Design review of the part built by this model. Coordinates are the model's own, in mm. Face numbers are marked on the shaded views. A direction names the side the tool comes from. Coordinates: 2 decimals unless noted, no trailing zeros. Order: outer loops, then holes, each group sorted by start corner. A loop starts at its lowest first (then second) coordinate and runs counter-clockwise, first axis right, second up.
from build123d import *

# Parameters (mm, degrees)
F0_W      = 9
F0_H      = 9
F1_DEPTH  = 4
F7_DEPTH  = 3.375
F8_DEPTH  = 3.375
F9_DEPTH  = 3.375
F10_DEPTH = 3.375
F11_D     = 13.25


with BuildPart() as f1:
    # F0 (on Top) → F1 (new body)
    with BuildSketch(Plane.XY):
        with BuildLine():
            ThreePointArc((4.5, -14.8323969742), (0, -15.5), (-4.5, -14.8323969742))
            Line((-4.5, -14.8323969742), (-4.5, -44.4))
            Line((-4.5, -44.4), (4.5, -44.4))
            Line((4.5, -44.4), (4.5, -14.8323969742))
        make_face()
        with BuildLine():
            Line((4.5, -4.5), (-4.5, -4.5))
            Line((-4.5, -4.5), (-4.5, -14.8323969742))
            ThreePointArc((-4.5, -14.8323969742), (0, -15.5), (4.5, -14.8323969742))
            Line((4.5, -14.8323969742), (4.5, -4.5))
        make_face()
        with BuildLine():
            Line((-4.5, -4.5), (-14.8323969742, -4.5))
            ThreePointArc((-14.8323969742, -4.5), (-10.9601551084, -10.9601551084), (-4.5, -14.8323969742))
            Line((-4.5, -14.8323969742), (-4.5, -4.5))
        make_face()
        with BuildLine():
            Line((-4.5, 4.5), (-14.8323969742, 4.5))
            ThreePointArc((-14.8323969742, 4.5), (-15.5, 0), (-14.8323969742, -4.5))
            Line((-14.8323969742, -4.5), (-4.5, -4.5))
            Line((-4.5, -4.5), (-4.5, 4.5))
        make_face()
        with BuildLine():
            Line((14.8323969742, -4.5), (4.5, -4.5))
            Line((4.5, -4.5), (4.5, -14.8323969742))
            ThreePointArc((4.5, -14.8323969742), (10.9601551084, -10.9601551084), (14.8323969742, -4.5))
        make_face()
        with BuildLine():
            Line((14.8323969742, 4.5), (4.5, 4.5))
            Line((4.5, 4.5), (4.5, -4.5))
            Line((4.5, -4.5), (14.8323969742, -4.5))
            ThreePointArc((14.8323969742, -4.5), (15.3321908594, -2.2746260022), (15.5, 0))
            ThreePointArc((15.5, 0), (15.3321908594, 2.2746260022), (14.8323969742, 4.5))
        make_face()
        with BuildLine():
            Line((44.4, 4.5), (14.8323969742, 4.5))
            ThreePointArc((14.8323969742, 4.5), (15.3321908594, 2.2746260022), (15.5, 0))
            ThreePointArc((15.5, 0), (15.3321908594, -2.2746260022), (14.8323969742, -4.5))
            Line((14.8323969742, -4.5), (44.4, -4.5))
            Line((44.4, -4.5), (44.4, 4.5))
        make_face()
        with BuildLine():
            Line((-14.8323969742, 4.5), (-44.4, 4.5))
            Line((-44.4, 4.5), (-44.4, -4.5))
            Line((-44.4, -4.5), (-14.8323969742, -4.5))
            ThreePointArc((-14.8323969742, -4.5), (-15.5, 0), (-14.8323969742, 4.5))
        make_face()
        Rectangle(F0_W, F0_H)
        with BuildLine():
            Line((-4.5, 14.8323969742), (-4.5, 4.5))
            Line((-4.5, 4.5), (4.5, 4.5))
            Line((4.5, 4.5), (4.5, 14.8323969742))
            ThreePointArc((4.5, 14.8323969742), (0, 15.5), (-4.5, 14.8323969742))
        make_face()
        with BuildLine():
            Line((4.5, 14.8323969742), (4.5, 4.5))
            Line((4.5, 4.5), (14.8323969742, 4.5))
            ThreePointArc((14.8323969742, 4.5), (10.9601551084, 10.9601551084), (4.5, 14.8323969742))
        make_face()
        with BuildLine():
            Line((-4.5, 44.4), (-4.5, 14.8323969742))
            ThreePointArc((-4.5, 14.8323969742), (0, 15.5), (4.5, 14.8323969742))
            Line((4.5, 14.8323969742), (4.5, 44.4))
            Line((4.5, 44.4), (-4.5, 44.4))
        make_face()
        with BuildLine():
            ThreePointArc((-4.5, 14.8323969742), (-10.9601551084, 10.9601551084), (-14.8323969742, 4.5))
            Line((-14.8323969742, 4.5), (-4.5, 4.5))
            Line((-4.5, 4.5), (-4.5, 14.8323969742))
        make_face()
    extrude(amount=F1_DEPTH)

    # F3 (on face) → F7 (join)
    with BuildSketch(Plane.XZ.offset(44.4)):
        with BuildLine():
            Line((4.5, 0), (-4.5, 0))
            Line((-4.5, 0), (-4.5, -3))
            ThreePointArc((-4.5, -3), (0, -1.5), (4.5, -3))
            Line((4.5, -3), (4.5, 0))
        make_face()
        with BuildLine():
            Line((4.5, -3), (-4.5, -3))
            ThreePointArc((-4.5, -3), (-7.4938552368, -9.3035353181), (-4, -15.3442887702))
            Line((-4, -15.3442887702), (-2.5, -10.4197270865))
            ThreePointArc((-2.5, -10.4197270865), (-0.7342087578, -6.2203305053), (2.875, -9))
            ThreePointArc((2.875, -9), (2.7796694947, -9.7342087578), (2.5, -10.4197270865))
            Line((2.5, -10.4197270865), (4, -15.3442887702))
            ThreePointArc((4, -15.3442887702), (6.5669627683, -12.6228441865), (7.5, -9))
            ThreePointArc((7.5, -9), (6.7082039325, -5.6458980338), (4.5, -3))
        make_face()
        with BuildLine():
            ThreePointArc((4.5, -3), (0, -1.5), (-4.5, -3))
            Line((-4.5, -3), (4.5, -3))
        make_face()
    extrude(amount=-F7_DEPTH)

    # F6 (on face) → F8 (join)
    with BuildSketch(Plane.YZ.offset(44.4)):
        with BuildLine():
            Line((4.5, 0), (-4.5, 0))
            Line((-4.5, 0), (-4.5, -3))
            ThreePointArc((-4.5, -3), (0, -1.5), (4.5, -3))
            Line((4.5, -3), (4.5, 0))
        make_face()
        with BuildLine():
            ThreePointArc((4.5, -3), (0, -1.5), (-4.5, -3))
            Line((-4.5, -3), (4.5, -3))
        make_face()
        with BuildLine():
            Line((4.5, -3), (-4.5, -3))
            ThreePointArc((-4.5, -3), (-7.4938552368, -9.3035353181), (-4, -15.3442887702))
            Line((-4, -15.3442887702), (-2.5, -10.4197270865))
            ThreePointArc((-2.5, -10.4197270865), (-0.7342087578, -6.2203305053), (2.875, -9))
            ThreePointArc((2.875, -9), (2.7796694947, -9.7342087578), (2.5, -10.4197270865))
            Line((2.5, -10.4197270865), (4, -15.3442887702))
            ThreePointArc((4, -15.3442887702), (6.5669627683, -12.6228441865), (7.5, -9))
            ThreePointArc((7.5, -9), (6.7082039325, -5.6458980338), (4.5, -3))
        make_face()
    extrude(amount=-F8_DEPTH)

    # F5 (on face) → F9 (join)
    with BuildSketch(Plane(origin=(0, 44.4, 0), x_dir=(-1, 0, 0), z_dir=(0, 1, 0))):
        with BuildLine():
            Line((4.5, 0), (-4.5, 0))
            Line((-4.5, 0), (-4.5, -3))
            ThreePointArc((-4.5, -3), (0, -1.5), (4.5, -3))
            Line((4.5, -3), (4.5, 0))
        make_face()
        with BuildLine():
            ThreePointArc((4.5, -3), (0, -1.5), (-4.5, -3))
            Line((-4.5, -3), (4.5, -3))
        make_face()
        with BuildLine():
            Line((4.5, -3), (-4.5, -3))
            ThreePointArc((-4.5, -3), (-7.4938552368, -9.3035353181), (-4, -15.3442887702))
            Line((-4, -15.3442887702), (-2.5, -10.4197270865))
            ThreePointArc((-2.5, -10.4197270865), (-0.7342087578, -6.2203305053), (2.875, -9))
            ThreePointArc((2.875, -9), (2.7796694947, -9.7342087578), (2.5, -10.4197270865))
            Line((2.5, -10.4197270865), (4, -15.3442887702))
            ThreePointArc((4, -15.3442887702), (6.5669627683, -12.6228441865), (7.5, -9))
            ThreePointArc((7.5, -9), (6.7082039325, -5.6458980338), (4.5, -3))
        make_face()
    extrude(amount=-F9_DEPTH)

    # F4 (on face) → F10 (join)
    with BuildSketch(Plane(origin=(-44.4, 0, 0), x_dir=(0, -1, 0), z_dir=(-1, 0, 0))):
        with BuildLine():
            Line((4.5, 0), (-4.5, 0))
            Line((-4.5, 0), (-4.5, -3))
            ThreePointArc((-4.5, -3), (0, -1.5), (4.5, -3))
            Line((4.5, -3), (4.5, 0))
        make_face()
        with BuildLine():
            Line((4.5, -3), (-4.5, -3))
            ThreePointArc((-4.5, -3), (-7.4938552368, -9.3035353181), (-4, -15.3442887702))
            Line((-4, -15.3442887702), (-2.5, -10.4197270865))
            ThreePointArc((-2.5, -10.4197270865), (-0.7342087578, -6.2203305053), (2.875, -9))
            ThreePointArc((2.875, -9), (2.7796694947, -9.7342087578), (2.5, -10.4197270865))
            Line((2.5, -10.4197270865), (4, -15.3442887702))
            ThreePointArc((4, -15.3442887702), (6.5669627683, -12.6228441865), (7.5, -9))
            ThreePointArc((7.5, -9), (6.7082039325, -5.6458980338), (4.5, -3))
        make_face()
        with BuildLine():
            ThreePointArc((4.5, -3), (0, -1.5), (-4.5, -3))
            Line((-4.5, -3), (4.5, -3))
        make_face()
    extrude(amount=-F10_DEPTH)

    # F11 (through all)
    with Locations(Plane(origin=(0, 0, 0), x_dir=(1, 0, 0), z_dir=(0, 0, -1))):
        with Locations((0, 0)):
            Hole(F11_D / 2)


solid = f1.part
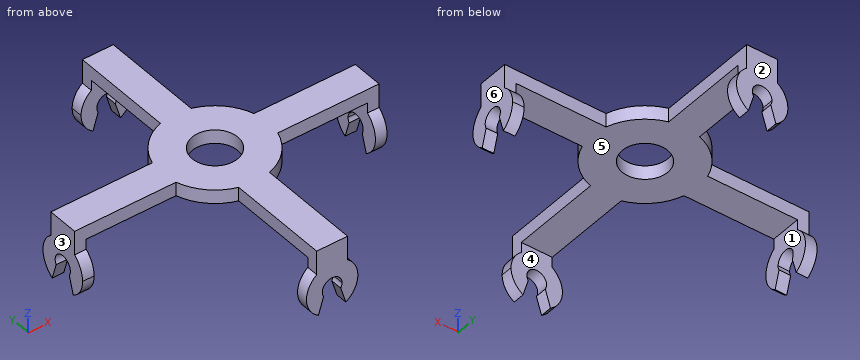
1. Mouldability with a two-part tool opening along X and no side actions: class the marked faces 1, 2 and 3 as pulls with the +X half, pulls with the -X half, needs draft (parallel to the pull), parting line crosses it, or undercut.
2. Add section A-A (y = 0). Give the boundary of the cut face in (x, z) (3 decimals), and give its area (3 significant figures).
3. For the marked faces 4, 5 and 6, list the 3-axis set-ups (+Z, -Z, +X, -X, +Y, -Y) from which the entire face can be reached by the end or side of a thin tool; tool diameter is ignored.
4. Add section D-D (x = 24.5). Give the boundary of the cut face in (y, z).
5. To check wall thickness, follow line 1 (Y direction, x = 7, z = -10.5) (3 decimals); line 2 (Y direction, x = -42.8, z = -9) (3 decimals). State the ranges of each line that lie inside material, in increasing order.
6. Insertion check: pin 1 (5.5 mm diameter, centred on y = -34.5, z = -0.5, fed in from -X); pin 2 (7.5 mm diameter, centred on y = 30, z = 2, fed in from +X); pin 3 (2 mm diameter, centred on y = -12.5, z = -2.5, fed in from +X); pin 4 (3.5 mm diameter, centred on x = 33, z = 1.5, fed in from -Y). Each pin has a flat end and moves straight along its axis. Give the tip position at first contact, or say it passes through.
7. Add section C-C (z = -12). State how many separate pieces and enclosed holes the cut face has, and give its area (3 significant figures).
Solution:
1. face 1: undercut
1. face 2: needs draft
1. face 3: pulls with the -X half
2. outline: (-44.4, -6.125) - (-41.025, -6.125) - (-41.025, 0) - (-6.625, 0) - (-6.625, 4) - (-44.4, 4) - close; (6.625, 0) - (41.025, 0) - (41.025, -6.125) - (44.4, -6.125) - (44.4, 4) - (6.625, 4) - close
2. area: 344 mm2
3. face 4: -Z, +X, -X
3. face 5: -Z
3. face 6: +Z, -Z, +X, +Y, -Y
4. outline: (-4.5, 0) - (4.5, 0) - (4.5, 4) - (-4.5, 4) - close
5. line 1: y = -44.4 to -41.025, 41.025 to 44.4
5. line 2: y = -7.5 to -2.875, 2.875 to 7.5
6. pin 1: stops at x = -4.5
6. pin 2: stops at x = 4.5
6. pin 3: passes through
6. pin 4: stops at y = -4.5
7. separate pieces: 8
7. enclosed holes: 0
7. area: 105 mm2
